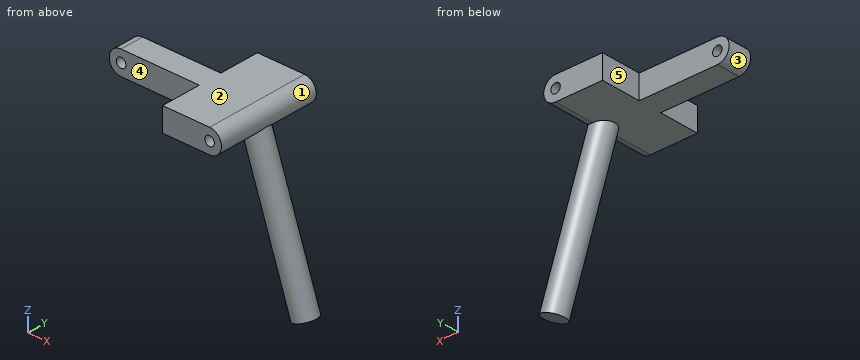
from build123d import *

# Parameters (mm, degrees)
BOSS_EXTRUDE1_DEPTH = 22
SKETCH2_R           = 1
CUT_EXTRUDE1_DEPTH  = 22
SKETCH3_W           = 5
SKETCH3_H           = 8.5
CUT_EXTRUDE7_DEPTH  = 19
BOSS_EXTRUDE3_START = -0.815625
SKETCH5_R           = 2.4
BOSS_EXTRUDE3_DEPTH = 32.815625


with BuildPart() as part:
    # Sketch1 → Boss-Extrude1 (new body)
    with BuildSketch(Plane(origin=(0, 0, 0), x_dir=(1, 0, 0), z_dir=(0, 1, 0))):
        with BuildLine():
            Line((0, 2.5), (26.41, 2.5))
            ThreePointArc((26.41, 2.5), (28.91, 0), (26.41, -2.5))
            Line((26.41, -2.5), (0, -2.5))
            ThreePointArc((0, -2.5), (-2.5, 0), (0, 2.5))
        make_face()
    extrude(amount=BOSS_EXTRUDE1_DEPTH)

    # Sketch2 → Cut-Extrude1 (cut)
    with BuildSketch(Plane(origin=(0, 22, 0), x_dir=(1, 0, 0), z_dir=(0, 1, 0))):
        Circle(SKETCH2_R)
        with Locations((26.41, 0)):
            Circle(SKETCH2_R)
    extrude(amount=-CUT_EXTRUDE1_DEPTH, mode=Mode.SUBTRACT)

    # Sketch3 → Cut-Extrude7 (cut)
    with BuildSketch(Plane(origin=(-2.5, 0, 0), x_dir=(0, 0, -1), z_dir=(1, 0, 0))):
        with Locations((0, 17.75)):
            Rectangle(SKETCH3_W, SKETCH3_H)
        with Locations((0, 4.25)):
            Rectangle(SKETCH3_W, SKETCH3_H)
    extrude(amount=CUT_EXTRUDE7_DEPTH, mode=Mode.SUBTRACT)

    # Sketch5 → Boss-Extrude3 (add)
    with BuildSketch(Plane(origin=(3.496027694, 0, -10.287166689), x_dir=(0, -1, 0), z_dir=(0.321769987, 0, -0.946817868)).offset(BOSS_EXTRUDE3_START)):
        with Locations((-11, -24.201034934)):
            Circle(SKETCH5_R)
    extrude(amount=BOSS_EXTRUDE3_DEPTH)


solid = part.part
Design review of the part built by this model. Coordinates are the model's own, in mm. Face numbers are marked on the shaded views. A direction names the side the tool comes from. Round coordinates to 2 decimals unless told otherwise and drop trailing zeros. Write each loop counter-clockwise with the first axis right and the second up, starting at its lowest first coordinate (ties: lowest second). Pieces come first, ordered by that corner, then holes.
Item 1: For the marked faces 1, 2, 3, 4 and 5, list the 3-axis set-ups (+Z, -Z, +X, -X, +Y, -Y) from which the entire face can be reached by the end or side of a thin tool; tool diameter is ignored.
Item 2: Consider section B-B on y = 7.25. Give the boundary of the cut face in (x, z), and give its area (3 significant figures).
Item 3: For pin 1 Ø2 at (y, z) = (6, -27.5) entering from -X; pin 2 Ø2 at (x, z) = (34, -27.5) entering from +Y; pin 3 Ø4 at (y, z) = (16.5, 1) entering from -X; pin 4 Ø6.5 at (x, y) = (9.5, 7.5) entering from -Z, all flat-tipped, find the tip position at first contact; note any pin that passes through.
Item 4: Wall thickness on L1, parallel to X at y = 11.75, z = 0; L2, parallel to Z at x = 26.41, y = 13.5; L3, parallel to Z at x = 12, y = 12: over which ranges is each line inside the solid? List them lowest first.
Item 5: Consider section C-C on x = 7.5. Give the boundary of the cut face in (y, z), and give its area (3 significant figures).
Item 6: Consider section A-A on z = 0. Give the boundary of the cut face in (x, y).
Check values:
1. face 1: +X
1. face 2: +Z, +X, -X, +Y, -Y
1. face 3: -X, +Y, -Y
1. face 4: +Z, -Z, -X, -Y
1. face 5: +Z, -Z, -X, +Y
2. outline: (16.5, -2.5) - (26.41, -2.5) arc R2.5 ccw to (26.41, 2.5) - (16.5, 2.5) - close; hole circle Ø2 at (26.41, 0)
2. area: 56.2 mm2
3. pin 1: passes through
3. pin 2: stops at y = 13.4
3. pin 3: stops at x = 16.5
3. pin 4: stops at z = -2.5
4. L1: x = -2.5 to -1, 1 to 25.41, 27.41 to 28.91
4. L2: z = -2.5 to -1, 1 to 2.5
4. L3: z = -2.5 to 2.5
5. outline: (8.5, -2.5) - (13.5, -2.5) - (13.5, 2.5) - (8.5, 2.5) - close
5. area: 25.0 mm2
6. outline: (-2.5, 8.5) - (-1, 8.5) - (-1, 13.5) - (-2.5, 13.5) - close; (1, 8.5) - (16.5, 8.5) - (16.5, 0) - (25.41, 0) - (25.41, 22) - (16.5, 22) - (16.5, 13.5) - (1, 13.5) - close; (27.41, 0) - (28.91, 0) - (28.91, 22) - (27.41, 22) - close
